Autodesk Inventor part; units mm, degrees
ref_plane "YZ Plane" through (0, 0, 0) normal (1, 0, 0) x (0, 1, 0)
ref_plane "XZ Plane" through (0, 0, 0) normal (0, 1, 0) x (-1, 0, 0)
ref_plane "XY Plane" through (0, 0, 0) normal (0, 0, 1) x (1, 0, 0)
sketch "Sketch1" plane through (0, 0, 0) normal (0, 0, 1) x (1, 0, 0)
  line L0 (-30, -30) -> (30, -30)
  line L1 (30, -30) -> (30, 30)
  line L2 (30, 30) -> (-30, 30)
  line L3 (-30, 30) -> (-30, -30)
  point P0 (0, 0)
  point P1 (-30, 0)
  point P2 (0, 30)
  dimension "d0" = 60
extrude "Extrusion1" add sketch "Sketch1" along normal blind 5
sketch "Sketch2" plane through (0, 0, 5) normal (0, 0, 1) x (1, 0, 0)
  line L0 (30, -30) -> (30, 30)
  line L1 (30, 1) -> (31, 1)
  line L2 (31, 1) -> (31, -1)
  line L3 (31, -1) -> (30, -1)
  line L4 (30, -1) -> (30, 1)
  point P0 (0, 0)
  point P1 (30, 0)
  point P2 (31, 0)
  dimension "d3" = 2
  dimension "d4" = 1
extrude "Extrusion2" add sketch "Sketch2" against normal up to surface (5 mm away)
pattern_circular "Circular Pattern1" count 4 over 360 about axis through (0, 0, -10) along (0, 0, 1) of "Extrusion2"
fillet "Fillet1" radius 4 4 edges at (30, -30, 2.5) (30, 30, 2.5) (-30, 30, 2.5) (-30, -30, 2.5)
shell "Shell1" thickness 2 removed faces 2 at (-0.3333, -9.3333, 5) at (-0.3333, -9.3333, 0)
sketch "Sketch3" plane through (0, 0, 0) normal (0, 0, -1) x (-1, 0, 0)
  arc A0 (30, 26) -> (26, 30) centre (26, 26) ccw
  line L0 (28.8284, 28.8284) -> (16.8284, 28.8284)
  line L1 (16.8284, 28.8284) -> (16.8284, 16.8284)
  line L2 (16.8284, 16.8284) -> (28.8284, 16.8284)
  line L3 (28.8284, 16.8284) -> (28.8284, 28.8284)
  point P0 (0, 0)
  dimension "d12" = 12
extrude "Extrusion3" add sketch "Sketch3" against normal blind 1
sketch "Sketch4" plane through (0, 0, 1) normal (0, 0, 1) x (1, 0, 0)
  arc A0 (-26, 28) -> (-28, 26) centre (-26, 26) ccw
  line L0 (-25, 25) -> (-22.4899, 25) construction
  line L1 (-22.4899, 25) -> (-22.4899, 17.9124) construction
  line L2 (-22.4899, 17.9124) -> (-25, 17.9124) construction
  line L3 (-25, 17.9124) -> (-25, 25) construction
  line L4 (-20.8039, 24.2901) -> (-23.5948, 24.2901)
  line L5 (-23.5948, 24.2901) -> (-23.5948, 22.5981)
  line L6 (-23.5948, 22.5981) -> (-20.9206, 22.5981)
  line L7 (-20.9206, 22.5981) -> (-20.9206, 21.8882)
  line L8 (-20.9206, 21.8882) -> (-23.5948, 21.8882)
  line L9 (-23.5948, 21.8882) -> (-23.5948, 19)
  line L10 (-23.5948, 19) -> (-24.3922, 19)
  line L11 (-24.3922, 19) -> (-24.3922, 25)
  line L12 (-24.3922, 25) -> (-20.8039, 25)
  line L13 (-20.8039, 25) -> (-20.8039, 24.2901)
  point P0 (0, 0)
  dimension "d15" = 1
  dimension "d16" = 1
emboss "Emboss1" sketch "Sketch4" operation add depth 1 direction (0, 0, -1)
properties part number "Jerk Store Test"
Work out the finished part from the listing and answer in its coordinate system (mm). A direction names the side the tool comes from. Round coordinates to 2 decimals unless told otherwise and drop trailing zeros. Loops run counter-clockwise (first coordinate to the right, second up) from the corner with the lowest first, then second, coordinate; pieces in that order, holes last. Notation, with made-up numbers: M 46.5,-11.5 L 101.5,-11.5 A24 ccw 101.5,5.5 Z; hole C 47,30 d3. An arc over 180 degrees is marked long. One line per question, with ' | ' between items.
Q1. Each of these flat-tipped pins is pushed along its axis until it touches: pin 1 Ø0.5 at (y, z) = (23.5, 1.5) entering from +X; pin 2 Ø0.8 at (x, z) = (-30.5, 2.5) entering from -Y; pin 3 Ø0.8 at (x, z) = (-22, 1.5) entering from -Y. Where does it stop, or does it pass through?
Conclusion:
pin 1: stops at x = 30 | pin 2: stops at y = -1 | pin 3: stops at y = -30
Q2. Find section B-B, the plane x = -19. Give the vertices of the cut face in (y, z), then the cut area to 3 significant figures.
Conclusion:
outline: M -30,0 L -28,0 L -28,5 L -30,5 Z; M 16.83,0 L 30,0 L 30,5 L 28,5 L 28,1 L 16.83,1 Z | area: 31.2 mm2
Q3. Consider line 1 along Y through (x, z) = (25, 1.3); line 2 along Y through (x, z) = (0.5, 0.3). Determine where each line is inside the solid, lowest interval first. Write a range as from..to.
Conclusion:
line 1: y = -30..-28, 28..30 | line 2: y = -31..-28, 28..31
Q4. The mould has two halves that part along X. Classify faces 6 (the flat face through (-14, -30, 2)), 7 (the flat face through (-31, 0, 3)), 8 (the cylindrical face through (-27.4, 27.43, 3.03)): +X half, -X half, draft (parallel to the pull), parting line (faces both ways), or undercut.
Conclusion:
face 6: draft | face 7: -X half | face 8: undercut
Q5. A tool of negligible diameter and unlimited length cuts with its end or side. For faces 1 (the flat face through (-13, 30, 2)), 2 (the cylindrical face through (-27.43, -27.4, 2.54)), 3 (the flat face through (30, -14, 2)), 4 (the flat face through (14, 30, 2)), 5 (the flat face through (-30, -13, 2)), from which of +Z, -Z, +X, -X, +Y, -Y can it reach the whole face along a straight path? Write none if from no direction.
Conclusion:
face 1: +Z, -Z, -X, +Y | face 2: +Z, -Z | face 3: +Z, -Z, +X, -Y | face 4: +Z, -Z, +X, +Y | face 5: +Z, -Z, -X, -Y
Q6. Find section A-A, the plane y = -17.5. Give the vertices of the cut face in (x, z).
Conclusion:
outline: M -30,0 L -28,0 L -28,5 L -30,5 Z; M 28,0 L 30,0 L 30,5 L 28,5 Z
